Design review of the part built by this model. Coordinates are the model's own, in mm. Face numbers are marked on the shaded views. A direction names the side the tool comes from. Coordinates: 2 decimals unless noted, no trailing zeros. Loops run counter-clockwise (first coordinate to the right, second up) from the corner with the lowest first, then second, coordinate; pieces in that order, holes last.
Q1. Add section D-D on z = 4.5. Give the boundary of the cut face in (x, y).
Q2. Draft analysis for pull direction Y (two halves, no side actions). For the marked faces 3, 4, 5 and 6, state which applies: released by +Y, released by -Y, zero draft, split by the parting line, or undercut.
Q3. Add section B-B on x = 1.5. Give the boundary of the cut face in (y, z), and give its area (3 significant figures).
Q4. For P1, Ø1.5, axis at x = 0.5, y = -5, coming from the +Z side, flat-tipped, find the tip position at first contact; note if it passes through.
Q5. Wall thickness on probe 1 along X at (y, z) = (1, 13.25); probe 2 along Y at (x, z) = (-0.25, 12); probe 3 along X at (y, z) = (9.25, 16): over which ranges is each line inside the solid? List them lowest first.
Q6. Machinability: for the marked faces 1 and 2, which of the approach directions +Z, -Z, +X, -X, +Y, -Y give a long, thin tool a straight path to every point of the face, cutting with its end or side? Answer none if there is none.
Q7. Add section A-A on z = 10.75. Give the boundary of the cut face in (x, y).
Q8. Add section C-C on y = -9. Give the boundary of the cut face in (x, z).
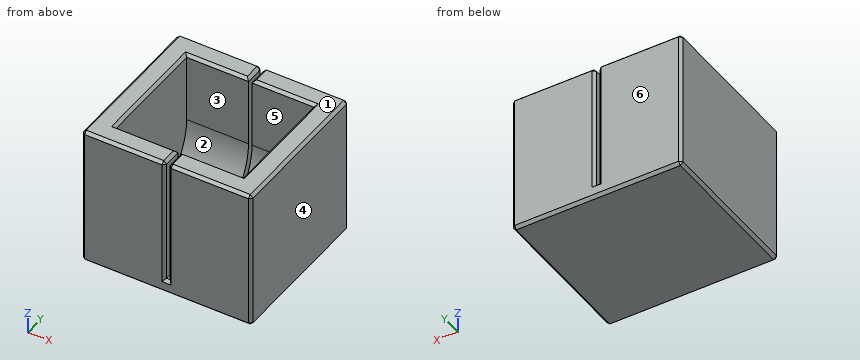
```python
from build123d import *

# Parameters (mm, degrees)
BOX002_W       = 0.5
BOX002_H       = 26
BOX002_DEPTH   = 24
CYLINDER_R     = 8
CYLINDER_DEPTH = 18
BOX001_W       = 18
BOX001_H       = 16
BOX001_DEPTH   = 10
BOX_W          = 24
BOX_H          = 22
BOX_DEPTH      = 20
CHAMFER_SIZE   = 0.4


with BuildPart() as cube002:
    # Box002 → Box002 (new body)
    with BuildSketch(Plane(origin=(-1.25, -13, 2), x_dir=(1, 0, 0), z_dir=(0, 0, 1))):
        with Locations((0.25, 13)):
            Rectangle(BOX002_W, BOX002_H)
    extrude(amount=BOX002_DEPTH)


with BuildPart() as cylinder:
    # Cylinder → Cylinder (new body)
    with BuildSketch(Plane(origin=(8, 0, 10), x_dir=(0, 0, 1), z_dir=(-1, 0, 0))):
        Circle(CYLINDER_R)
    extrude(amount=CYLINDER_DEPTH)


with BuildPart() as fusion:
    # Box001 → Box001 (new body)
    with BuildSketch(Plane(origin=(-10, -8, 10), x_dir=(1, 0, 0), z_dir=(0, 0, 1))):
        with Locations((9, 8)):
            Rectangle(BOX001_W, BOX001_H)
    extrude(amount=BOX001_DEPTH)

    # Fusion: union Cylinder
    add(cylinder.part)


with BuildPart() as chamfer_body:
    # Box → Box (new body)
    with BuildSketch(Plane(origin=(-13, -11, 0), x_dir=(1, 0, 0), z_dir=(0, 0, 1))):
        with Locations((12, 11)):
            Rectangle(BOX_W, BOX_H)
    extrude(amount=BOX_DEPTH)

    # Cut: cut Fusion
    add(fusion.part, mode=Mode.SUBTRACT)

    # Cut001: cut Cube002
    add(cube002.part, mode=Mode.SUBTRACT)

    # Chamfer
    chamfer_edges = [chamfer_body.edges().sort_by_distance(p)[0] for p in [
        (-13, -11, 10),
        (-13, 0, 20),
        (-13, 11, 10),
        (-13, 0, 0),
        (11, -11, 10),
        (5.125, -11, 20),
        (-0.75, -11, 11),
        (-1, -11, 2),
        (-1.25, -11, 11),
        (-7.125, -11, 20),
        (-1, -11, 0),
        (-7.125, 11, 20),
        (-1.25, 9.5, 20),
        (-5.625, 8, 20),
        (-10, 0, 20),
        (-5.625, -8, 20),
        (-1.25, -9.5, 20),
        (11, 11, 10),
        (5.125, 11, 20),
        (-0.75, 11, 11),
        (-1, 11, 2),
        (-1.25, 11, 11),
        (-1, 11, 0),
        (11, 0, 0),
        (11, 0, 20),
        (-0.75, -9.5, 20),
        (3.625, -8, 20),
        (8, 0, 20),
        (3.625, 8, 20),
        (-0.75, 9.5, 20),
    ]]
    chamfer(chamfer_edges, length=CHAMFER_SIZE)


solid = chamfer_body.part
```
Entries:
1. outline: (-13, -10.6) - (-12.6, -11) - (-1.65, -11) - (-1.25, -10.6) - (-1.25, -5.81) - (-10, -5.81) - (-10, 5.81) - (-1.25, 5.81) - (-1.25, 10.6) - (-1.65, 11) - (-12.6, 11) - (-13, 10.6) - close; (-0.75, -10.6) - (-0.35, -11) - (10.6, -11) - (11, -10.6) - (11, 10.6) - (10.6, 11) - (-0.35, 11) - (-0.75, 10.6) - (-0.75, 5.81) - (8, 5.81) - (8, -5.81) - (-0.75, -5.81) - close
2. face 3: undercut
2. face 4: zero draft
2. face 5: undercut
2. face 6: released by +Y
3. outline: (-11, 0.4) - (-10.6, 0) - (10.6, 0) - (11, 0.4) - (11, 19.6) - (10.6, 20) - (8.4, 20) - (8, 19.6) - (8, 10) arc R8 cw to (-8, 10) - (-8, 19.6) - (-8.4, 20) - (-10.6, 20) - (-11, 19.6) - close
3. area: 179 mm2
4. P1: stops at z = 4.44
5. probe 1: x = -13 to -10, 8 to 11
5. probe 2: y = -11 to -8, 8 to 11
5. probe 3: x = -13 to -1.25, -0.75 to 11
6. face 1: +Z, +X, -X, +Y, -Y
6. face 2: +Z
7. outline: (-13, -10.6) - (-12.6, -11) - (-1.65, -11) - (-1.25, -10.6) - (-1.25, -8) - (-10, -8) - (-10, 8) - (-1.25, 8) - (-1.25, 10.6) - (-1.65, 11) - (-12.6, 11) - (-13, 10.6) - close; (-0.75, -10.6) - (-0.35, -11) - (10.6, -11) - (11, -10.6) - (11, 10.6) - (10.6, 11) - (-0.35, 11) - (-0.75, 10.6) - (-0.75, 8) - (8, 8) - (8, -8) - (-0.75, -8) - close
8. outline: (-13, 0.4) - (-12.6, 0) - (10.6, 0) - (11, 0.4) - (11, 19.6) - (10.6, 20) - (-0.35, 20) - (-0.75, 19.6) - (-0.75, 2) - (-1.25, 2) - (-1.25, 19.6) - (-1.65, 20) - (-12.6, 20) - (-13, 19.6) - close
